```python
from build123d import *

# Parameters (mm, degrees)
SKETCH1_W           = 25
SKETCH1_H           = 23
BOSS_EXTRUDE1_DEPTH = 15
SHELL1_T            = -1.5
SKETCH3_W           = 2
SKETCH3_H           = 2
BOSS_EXTRUDE2_DEPTH = 2
SKETCH4_W           = 2
SKETCH4_H           = 7
BOSS_EXTRUDE3_DEPTH = 2
SKETCH5_W           = 10
SKETCH5_H           = 3
BOSS_EXTRUDE4_DEPTH = 10
SKETCH2_R           = 1.75
BOSS_EXTRUDE5_DEPTH = 2
SKETCH6_R           = 1.25
BOSS_EXTRUDE6_DEPTH = 4


with BuildPart() as part:
    # Sketch1 → Boss-Extrude1 (new body)
    with BuildSketch(Plane(origin=(0, 0, 0), x_dir=(1, 0, 0), z_dir=(0, 1, 0))):
        Rectangle(SKETCH1_W, SKETCH1_H)
    extrude(amount=BOSS_EXTRUDE1_DEPTH)

    # Shell1
    shell1_openings = [part.faces().sort_by_distance(p)[0] for p in [
        (0, 15, 0),
    ]]
    offset(amount=SHELL1_T, openings=shell1_openings, kind=Kind.INTERSECTION)

    # Sketch3 → Boss-Extrude2 (add)
    with BuildSketch(Plane(origin=(0, 1.5, 0), x_dir=(1, 0, 0), z_dir=(0, 1, 0))):
        with Locations((-10, 9)):
            Rectangle(SKETCH3_W, SKETCH3_H)
        with Locations((10, 9)):
            Rectangle(SKETCH3_W, SKETCH3_H)
        with Locations((10, -9)):
            Rectangle(SKETCH3_W, SKETCH3_H)
        with Locations((-10, -9)):
            Rectangle(SKETCH3_W, SKETCH3_H)
    extrude(amount=BOSS_EXTRUDE2_DEPTH)

    # Sketch4 → Boss-Extrude3 (add)
    with BuildSketch(Plane(origin=(0, 1.5, 0), x_dir=(1, 0, 0), z_dir=(0, 1, 0))):
        with Locations((-10, 4.5)):
            Rectangle(SKETCH4_W, SKETCH4_H)
        with Locations((10, 4.5)):
            Rectangle(SKETCH4_W, SKETCH4_H)
    extrude(amount=BOSS_EXTRUDE3_DEPTH)

    # Sketch5 → Boss-Extrude4 (add)
    with BuildSketch(Plane(origin=(0, 1.5, 0), x_dir=(1, 0, 0), z_dir=(0, 1, 0))):
        with Locations((-6, 8.5)):
            Rectangle(SKETCH5_W, SKETCH5_H)
    extrude(amount=BOSS_EXTRUDE4_DEPTH)

    # Sketch2 → Boss-Extrude5 (add)
    with BuildSketch(Plane(origin=(0, 1.5, 0), x_dir=(1, 0, 0), z_dir=(0, 1, 0))):
        with Locations((-8.2, -7.25)):
            Circle(SKETCH2_R)
        with Locations((8.2, -7.25)):
            Circle(SKETCH2_R)
    extrude(amount=BOSS_EXTRUDE5_DEPTH)

    # Sketch6 → Boss-Extrude6 (add)
    with BuildSketch(Plane(origin=(0, 3.5, 0), x_dir=(1, 0, 0), z_dir=(0, 1, 0))):
        with Locations((-8.2, -7.25)):
            Circle(SKETCH6_R)
        with Locations((8.2, -7.25)):
            Circle(SKETCH6_R)
    extrude(amount=BOSS_EXTRUDE6_DEPTH)


solid = part.part
```
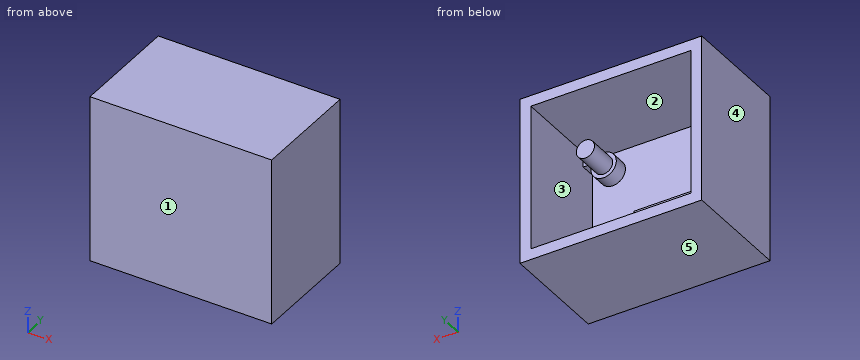
For this review, take the finished solid that the model builds, in its own axes (mm). Face numbers are marked on the shaded views. A direction names the side the tool comes from. Give positions to 0.01 mm unless a question says otherwise; leave off trailing zeros. Write each loop counter-clockwise with the first axis right and the second up, starting at its lowest first coordinate (ties: lowest second). Pieces come first, ordered by that corner, then holes.
Item 1: Take a section at B-B (y = 2). Give the boundary of the cut face in (x, z), and give its area (3 significant figures).
Item 2: The part is to be moulded in two halves that separate along X. For the marked faces 3, 4 and 5, say which applies: +X half, -X half, draft (parallel to the pull), parting line (faces both ways), or undercut.
Item 3: Machinability: for the marked faces 1 and 2, which of the approach directions +Z, -Z, +X, -X, +Y, -Y give a long, thin tool a straight path to every point of the face, cutting with its end or side? Answer none if there is none.
Item 4: Wall thickness on probe 1 along X at (y, z) = (7.5, 1); probe 2 along Z at (x, y) = (-5, 7); probe 3 along Z at (x, y) = (3.25, 5.5): over which ranges is each line inside the solid? List them lowest first.
Item 5: Take a section at D-D (y = 10.5). Give the boundary of the cut face in (x, z), and give its area (3 significant figures).
Item 6: Insertion check: P1, Ø2, axis at x = -8.5, z = 7, coming from the +Y side. The pin has a flat end and moves straight along its axis. Give the tip position at first contact, or say it passes through.
Item 7: Take a section at A-A (x = -3.25). Give the boundary of the cut face in (y, z).
Item 8: Take a section at C-C (z = 7.25). Give the boundary of the cut face in (x, y).
Established:
1. outline: (-12.5, -11.5) - (12.5, -11.5) - (12.5, 11.5) - (-12.5, 11.5) - close; hole (-11, -1) - (-9, -1) - (-9, -7) - (-1, -7) - (-1, -10) - (9, -10) - (9, -1) - (11, -1) - (11, 8) - (9.78, 8) arc R1.75 cw (long way) to (9, 8.81) - (9, 10) - (-9, 10) - (-9, 8.81) arc R1.75 cw (long way) to (-9.78, 8) - (-11, 8) - close
1. area: 221 mm2
2. face 3: undercut
2. face 4: -X half
2. face 5: draft
3. face 1: +Z, -Z, +X, -X, -Y
3. face 2: +Y
4. probe 1: x = -12.5 to -11, 11 to 12.5
4. probe 2: z = -11.5 to -7, 10 to 11.5
4. probe 3: z = -11.5 to -10, 10 to 11.5
5. outline: (-12.5, -11.5) - (12.5, -11.5) - (12.5, 11.5) - (-12.5, 11.5) - close; hole (-11, -7) - (-1, -7) - (-1, -10) - (11, -10) - (11, 10) - (-11, 10) - close
5. area: 165 mm2
6. P1: stops at y = 7.5
7. outline: (0, -11.5) - (15, -11.5) - (15, -10) - (11.5, -10) - (11.5, -7) - (1.5, -7) - (1.5, 10) - (15, 10) - (15, 11.5) - (0, 11.5) - close
8. outline: (-12.5, 0) - (12.5, 0) - (12.5, 15) - (11, 15) - (11, 1.5) - (9.95, 1.5) - (9.95, 3.5) - (9.45, 3.5) - (9.45, 7.5) - (6.95, 7.5) - (6.95, 3.5) - (6.45, 3.5) - (6.45, 1.5) - (-6.45, 1.5) - (-6.45, 3.5) - (-6.95, 3.5) - (-6.95, 7.5) - (-9.45, 7.5) - (-9.45, 3.5) - (-9.95, 3.5) - (-9.95, 1.5) - (-11, 1.5) - (-11, 15) - (-12.5, 15) - close
